The model under review builds one solid part; all positions refer to its coordinate system, in mm. Face numbers are marked on the shaded views. A direction names the side the tool comes from. Give positions to 0.01 mm unless a question says otherwise; leave off trailing zeros. Loops run counter-clockwise (first coordinate to the right, second up) from the corner with the lowest first, then second, coordinate; pieces in that order, holes last. Notation, with made-up numbers: (78.5, -36.75) - (137.5, -36.75) arc R9 cw to (137.5, -23.75) - close; hole circle Ø10 at (-34, 48). An arc over 180 degrees is marked (long way). Answer as a JSON object with one key per item and string values.
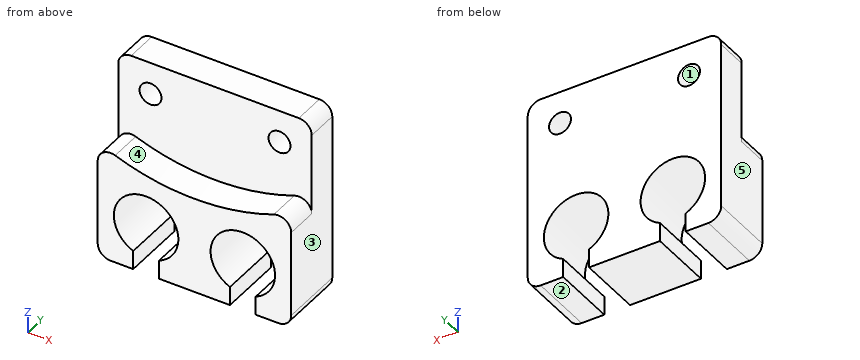
Autodesk Inventor part; units mm, degrees
ref_plane "YZ Plane" through (0, 0, 0) normal (1, 0, 0) x (0, 1, 0)
ref_plane "XZ Plane" through (0, 0, 0) normal (0, 1, 0) x (-1, 0, 0)
ref_plane "XY Plane" through (0, 0, 0) normal (0, 0, 1) x (1, 0, 0)
sketch "スケッチ1" plane through (0, 0, 0) normal (0, 1, 0) x (-1, 0, 0)
  line L0 (15, 10) -> (-15, 10)
  line L1 (-15, 10) -> (-15, -20)
  line L2 (-15, -20) -> (15, -20)
  line L3 (15, -20) -> (15, 10)
  line L4 (15, 10) -> (-15, -20) construction
  line L5 (-15, 10) -> (15, -20) construction
  point P0 (0, 0)
  point P1 (0, -5)
  dimension "d0" = 30
  dimension "d15" = 10
  dimension "d16" = 20
extrude "押し出し1" add sketch "スケッチ1" along normal mid plane 10
sketch "スケッチ2" plane through (0, 5, 0) normal (0, 1, 0) x (1, 0, 0)
  line L0 (-15, -10) -> (15, -10)
  point P0 (0, 0)
  point P1 (-10, -5)
  point P2 (10, -5)
  dimension "d4" = 10
  dimension "d5" = 10
  dimension "d6" = 5
hole "穴1" at (-10, 5, 5) at (10, 5, 5) direction (0, -1, 0) diameter 3.4 end through all
sketch "スケッチ3" plane through (0, -5, 0) normal (0, -1, 0) x (1, 0, 0)
  circle A0 centre (0, 30) radius 34.9965
  circle A1 centre (-10, 5) radius 1.7
  point P0 (0, 0)
  dimension "d17" = 25
  dimension "d18" = 69.993
extrude "押し出し2" cut sketch "スケッチ3" against normal blind 5
fillet "フィレット1" radius 2 2 edges at (15, -2.5, -1.6189) (-15, -2.5, -1.6189)
fillet "フィレット2" radius 2 2 edges at (15, 2.5, 10) (-15, 2.5, 10)
fillet "フィレット3" radius 2 2 edges at (15, 0, -20) (-15, 0, -20)
sketch "スケッチ4" plane through (0, 5, 0) normal (0, 1, 0) x (1, 0, 0)
  circle A0 centre (-7.5, 12.5) radius 5
  circle A1 centre (7.5, 12.5) radius 5
  line L0 (13, 20) -> (-13, 20)
  line L1 (-15, 18) -> (-15, -8)
  line L2 (15, -8) -> (15, 18)
  point P0 (0, 0)
  dimension "d26" = 10
  dimension "d27" = 10
  dimension "d28" = 7.5
  dimension "d29" = 7.5
  dimension "d30" = 7.5
  dimension "d31" = 7.5
extrude "押し出し3" cut sketch "スケッチ4" against normal through all
sketch "スケッチ5" plane through (0, 5, 0) normal (0, 1, 0) x (1, 0, 0)
  circle A0 centre (-7.5, 12.5) radius 5
  circle A1 centre (7.5, 12.5) radius 5
  line L0 (-9.5, 17.0826) -> (-5.5, 17.0826)
  line L1 (-5.5, 17.0826) -> (-5.5, 20)
  line L2 (-5.5, 20) -> (-9.5, 20)
  line L3 (-9.5, 20) -> (-9.5, 17.0826)
  line L4 (-9.5, 17.0826) -> (-5.5, 20) construction
  line L5 (-5.5, 17.0826) -> (-9.5, 20) construction
  line L6 (5.5, 17.0826) -> (9.5, 17.0826)
  line L7 (9.5, 17.0826) -> (9.5, 20)
  line L8 (9.5, 20) -> (5.5, 20)
  line L9 (5.5, 20) -> (5.5, 17.0826)
  line L10 (5.5, 17.0826) -> (9.5, 20) construction
  line L11 (9.5, 17.0826) -> (5.5, 20) construction
  line L12 (13, 20) -> (-13, 20)
  point P0 (0, 0)
  point P1 (-7.5, 18.5413)
  point P2 (7.5, 18.5413)
  point P3 (-7.5, 18.5413)
  point P4 (7.5, 18.5413)
  dimension "d34" = 4
  dimension "d35" = 4
extrude "押し出し4" cut sketch "スケッチ5" against normal through all contours L8 L7 A1 L9 | L0 A0 | A0 L3 L2 L1 | A1 L6 picked at (-7.8405, 17.1866) picked at (7.1595, 17.1866)
equation "\"d29\" = d28"
equation "\"d30\" = d28"
equation "\"d31\" = d29"
equation "\"d35\" = d34"
properties part number "scara-base11" material "ABS プラスチック"
Q1. Consider section C-C, the plane x = 10. State the section outline as (y, z) points.
Results:
{"outline": "(-5, -20) - (5, -20) - (5, -16.83) - (-5, -16.83) - close; (-5, -8.17) - (5, -8.17) - (5, 3.3) - (0, 3.3) - (0, -3.54) - (-5, -3.54) - close; (0, 6.7) - (5, 6.7) - (5, 10) - (0, 10) - close"}
Q2. Clearance check with flat-ended pins moving along their axes: pin 1 Ø0.9 at (y, z) = (-1, -19) entering from +X; pin 2 Ø2.5 at (x, z) = (-10, 5) entering from +Y; pin 3 Ø4 at (x, z) = (10, 5) entering from -Y; pin 4 Ø8 at (x, z) = (9.5, -12.5) entering from -Y. State where each tip first meets the part, or that it passes through.
Results:
{"pin 1": "stops at x = 14.92", "pin 2": "passes through", "pin 3": "stops at y = 0", "pin 4": "stops at y = -5"}
Q3. Consider section D-D, the plane y = -3. State the section outline as (x, z) points.
Results:
{"outline": "(-15, -18) arc R2 ccw to (-13, -20) - (-9.5, -20) - (-9.5, -17.08) arc R5 cw (long way) to (-5.5, -17.08) - (-5.5, -20) - (5.5, -20) - (5.5, -17.08) arc R5 cw (long way) to (9.5, -17.08) - (9.5, -20) - (13, -20) arc R2 ccw to (15, -18) - (15, -4.64) arc R2 ccw to (12.3, -2.76) arc R35 cw to (-12.3, -2.76) arc R2 ccw to (-15, -4.64) - close"}
Q4. To check wall thickness, follow probe 1 along X at (y, z) = (3.5, 5); probe 2 along X at (y, z) = (-2, -12.5); probe 3 along Y at (x, z) = (2.5, 5). State the ranges of each line that lie inside material, in increasing order. Write a range as [from, to].
Results:
{"probe 1": "x = [-15, -11.7], [-8.3, 8.3], [11.7, 15]", "probe 2": "x = [-15, -12.5], [-2.5, 2.5], [12.5, 15]", "probe 3": "y = [0, 5]"}
Q5. Consider section B-B, the plane y = 1.75. State the section outline as (x, z) points.
Results:
{"outline": "(-15, -18) arc R2 ccw to (-13, -20) - (-9.5, -20) - (-9.5, -17.08) arc R5 cw (long way) to (-5.5, -17.08) - (-5.5, -20) - (5.5, -20) - (5.5, -17.08) arc R5 cw (long way) to (9.5, -17.08) - (9.5, -20) - (13, -20) arc R2 ccw to (15, -18) - (15, 8) arc R2 ccw to (13, 10) - (-13, 10) arc R2 ccw to (-15, 8) - close; hole circle Ø3.4 at (-10, 5); hole circle Ø3.4 at (10, 5)"}
Q6. For the marked faces 4 and 5, list the 3-axis set-ups (+Z, -Z, +X, -X, +Y, -Y) from which the entire face can be reached by the end or side of a thin tool; tool diameter is ignored.
Results:
{"face 4": "+Z, -Y", "face 5": "+Z, -Z, -X, +Y, -Y"}
Q7. The part is to be moulded in two halves that separate along X. For the marked faces 1, 2 and 3, say which applies: +X half, -X half, draft (parallel to the pull), parting line (faces both ways), or undercut.
Results:
{"face 1": "undercut", "face 2": "draft", "face 3": "+X half"}
Q8. Consider section A-A, the plane z = 5. State the section outline as (x, y) points, plus the area to 3 significant figures.
Results:
{"outline": "(-15, 0) - (-11.7, 0) - (-11.7, 5) - (-15, 5) - close; (-8.3, 0) - (8.3, 0) - (8.3, 5) - (-8.3, 5) - close; (11.7, 0) - (15, 0) - (15, 5) - (11.7, 5) - close", "area": "116 mm^2"}
